Source: CAD feature listing. Evaluate the final solid. Frame: model axes, mm. Coordinates: 2 decimals unless noted, no trailing zeros. Order: outer loops, then holes, each group sorted by start corner. A loop starts at its lowest first (then second) coordinate and runs counter-clockwise, first axis right, second up. Notation, with made-up numbers: (72.5, 60.25) - (126.5, 60.25) arc R5 cw to (126.5, 65.25) - close; hole circle Ø2 at (83.5, 57.25). An arc over 180 degrees is marked (long way). One line per question, with ' | ' between items. Start each with the question number.
(1) Section A-A (z = 1.95). Return the cut outline in (x, y).
(2) Contact query for a flat-ended pin moving along its axis: P1, Ø1, axis at x = 9, z = 0.5, coming from the +Y side. Output: stop coordinate, or through.
(3) Line query: line 1 along X through (y, z) = (26.5, 0.4); line 2 along Y through (x, z) = (8, 3.1); line 3 along Y through (x, z) = (7.5, 2.55). Output: solid intervals per line, ascending.
(4) Section B-B (y = 30). Return the cut outline in (x, z), then the cut area to 3 significant figures.
(5) Section C-C (x = -2). Return the cut outline in (y, z), then the cut area to 3 significant figures.
from build123d import *

# Parameters (mm, degrees)
F1_DEPTH    = 0.508
F2_DEPTH    = 3.048
F3_T1_DEPTH = 47.7471989741
F3_T3_DEPTH = 47.4709696523
F3_T5_DEPTH = 47.6607350592
F3_T7_DEPTH = 46.5501838511
F3_T9_DEPTH = 46.8386979916


# Not quite as in the source:
# - a fillet or chamfer that OpenCascade refuses, or shapes differently, is made with other operations: its cross-section is extruded or revolved along the edge and cut away or added


with BuildPart() as f1:
    # F0 (on Top) → F1 (new body)
    with BuildSketch(Plane.XY):
        Polygon((-17.6225993782, 12.5228120014), (0, 0), (17.2826144844, 12.5228120014), (17.2826144844, 34.0552479029), (0, 44.934798032), (-17.6225993782, 34.0552479029), align=None)
    extrude(amount=F1_DEPTH)

    # F2 (add): a face of the model
    f2_faces = [f1.faces().sort_by_distance(p)[0] for p in [
        (-0.1500416402, 22.8299999891, 0.508),
    ]]
    extrude(f2_faces, amount=F2_DEPTH)

    # F3: chamfer of 5.08 on 6 edges, made by hand

    # F3_s2 → F3_t1 (cut)
    with BuildSketch(Plane(origin=(-28.2718126223, 20.0902594906, 0), x_dir=(0, 0, 1), z_dir=(0.8151478349, -0.5792529735, 0))):
        Polygon((-1.524, 0), (3.556, -5.08), (3.556, 0), align=None)
    extrude(amount=F3_T1_DEPTH, mode=Mode.SUBTRACT)

    # F3_s4 → F3_t3 (cut)
    with BuildSketch(Plane(origin=(-10.5789320411, -7.6653898197, 0), x_dir=(0, 0, 1), z_dir=(0.8097681351, 0.5867500042, 0))):
        Polygon((-1.524, 0), (3.556, -5.08), (3.556, 0), align=None)
    extrude(amount=F3_T3_DEPTH, mode=Mode.SUBTRACT)

    # F3_s6 → F3_t5 (cut)
    with BuildSketch(Plane.XZ.offset(-47.1193974817)):
        Polygon((17.2826144844, -1.524), (12.2026144844, 3.556), (17.2826144844, 3.556), align=None)
        Polygon((-12.5425993782, 3.556), (-17.6225993782, -1.524), (-17.6225993782, 3.556), align=None)
    extrude(amount=F3_T5_DEPTH, mode=Mode.SUBTRACT)

    # F3_s8 → F3_t7 (cut)
    with BuildSketch(Plane(origin=(8.0798332195, -5.0863224789, 0), x_dir=(0, 0, 1), z_dir=(-0.846279114, 0.5327397688, 0))):
        Polygon((-1.524, 38.0273810661), (3.556, 32.9473810661), (3.556, 38.0273810661), align=None)
    extrude(amount=F3_T7_DEPTH, mode=Mode.SUBTRACT)

    # F3_s10 → F3_t9 (cut)
    with BuildSketch(Plane(origin=(31.2020521098, 19.2630089793, 0), x_dir=(0, 0, 1), z_dir=(-0.850905843, -0.5253182334, 0))):
        Polygon((-1.524, 38.2352821986), (3.556, 33.1552821986), (3.556, 38.2352821986), align=None)
    extrude(amount=F3_T9_DEPTH, mode=Mode.SUBTRACT)


solid = f1.part
Response values:
1) outline: (-14.15, 14.32) - (-0.02, 4.28) - (13.81, 14.3) - (13.81, 32.14) - (-0.02, 40.84) - (-14.15, 32.12) - close
2) P1: stops at y = 37.55
3) line 1: x = -15.7 to 15.36 | line 2: y = 11.51 to 34.43 | line 3: y = 10.47 to 35.4
4) outline: (-16.1, 0) - (15.76, 0) - (12.2, 3.56) - (-12.54, 3.56) - close | area: 101 mm²
5) outline: (3.29, 0) - (41.91, 0) - (37.73, 3.56) - (7.65, 3.56) - close | area: 122 mm²
